Work out the finished part from the listing and answer in its coordinate system (mm). Face numbers are marked on the shaded views. A direction names the side the tool comes from. Round coordinates to 2 decimals unless told otherwise and drop trailing zeros. Write each loop counter-clockwise with the first axis right and the second up, starting at its lowest first coordinate (ties: lowest second). Pieces come first, ordered by that corner, then holes. Notation, with made-up numbers: (24, 45) -> (64, 45) arc R31 ccw to (64, 70) -> close; hole circle Ø9 at (54, -37.5). An arc over 180 degrees is marked (long way). One line per question, with ' | ' between items. Start each with the question number.
Autodesk Fusion 360 part; units mm, degrees
sketch "Sketch1" plane through (0, 0, 0) normal (0, 0, 1) x (1, 0, 0)
  line L0 (0, 0) -> (33, 0)
  line L1 (33, 0) -> (33, -45)
  line L2 (33, -45) -> (0, -45)
  line L3 (0, -45) -> (0, 0)
  circle A0 centre (31, -2) radius 1
  circle A1 centre (2, -2) radius 1
  circle A2 centre (2, -43) radius 1
  circle A3 centre (31, -43) radius 1
  line L4 (34, 1) -> (34, -46)
  line L5 (34, -46) -> (-1, -46)
  line L6 (-1, -46) -> (-1, 1)
  line L7 (-1, 1) -> (34, 1)
  line L8 (36, 3) -> (36, -48)
  line L9 (36, -48) -> (-3, -48)
  line L10 (-3, -48) -> (-3, 3)
  line L11 (-3, 3) -> (36, 3)
  circle A4 centre (31, -2) radius 2
  circle A5 centre (31, -43) radius 2
  circle A6 centre (2, -43) radius 2
  circle A7 centre (2, -2) radius 2
  line L12 (31, -36) -> (2, -36)
  line L13 (2, -36) -> (2, -7)
  line L14 (2, -7) -> (31, -7)
  line L15 (31, -7) -> (31, -36)
extrude "Extrude1" add sketch "Sketch1" along normal blind 20 contours L8 L9 L10 L11 makes body 1
extrude "Extrude2" add sketch "Sketch1" along normal blind 4 separate body contours A7 | A4 | A6 | A5 makes body 2 at (32.9975, -43.0997, 1.3333) makes body 3 at (0.6766, -41.5004, 2.6667) makes body 4 at (32.9975, -2.0997, 1.3333) makes body 5 at (3.9975, -2.0997, 1.3333)
extrude "Extrude3" add sketch "Sketch1" against normal blind 1 contours L0 L3 A7 | L0 L1 L2 L3 A4 A5 A6 A7 | A7 | L0 L1 A4 | A4 | L2 L3 A6 | A6 | A5 | L1 L2 A5 | A0 | A1 | A2 | A3 | L4 L5 L6 L7 | L8 L9 L10 L11 bodies 1 2 3 4 5
extrude "Extrude4" cut 1 faces at (35.3333, -30.3333, 20) along direction (0, 0, -1) blind 10 on bodies 1 bodies 1
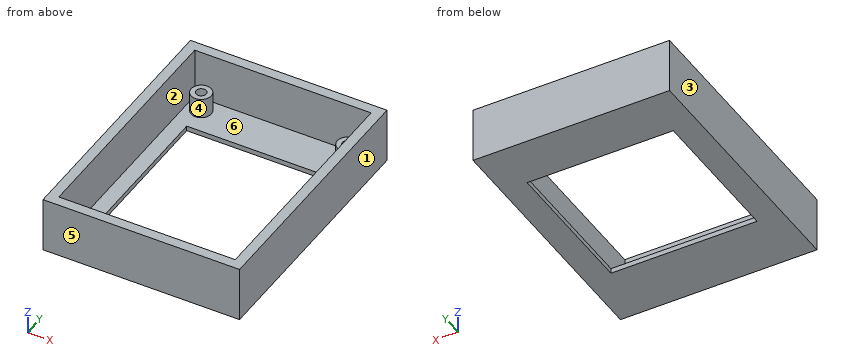
(1) A cutting plane is placed at D-D, the plane z = 6.75. Determine the outline of the cut face in (x, y).
(2) Given pin 1 Ø0.6 at (x, y) = (31, -43) entering from +Z; pin 2 Ø1.2 at (x, y) = (1.5, -1.5) entering from +Z; pin 3 Ø10 at (x, y) = (30, -37) entering from +Z, each flat-ended and moving along its own axis, determine where each tip first touches the part or whether it passes through.
(3) A cutting plane is placed at C-C, the plane x = 19. Determine the outline of the cut face in (y, z), then the cut area to 3 significant figures.
(4) A cutting plane is placed at A-A, the plane y = -29. Determine the outline of the cut face in (x, z).
(5) A cutting plane is placed at B-B, the plane z = 2.75. Count the separate pieces of the cut face and the enclosed holes in it, then the cut area to 3 significant figures.
(6) The mould has two halves that part along X. Classify the marked faces 3, 4, 5 and 6: +X half, -X half, draft (parallel to the pull), parting line (faces both ways), or undercut.
(7) Consider L1, parallel to Y at x = 31, z = 2.4; L2, parallel to X at y = -35, z = 3; L3, parallel to Y at x = 30, z = 4.25. Determine where each line is inside the solid, lowest interval first.
(8) For the marked faces 1 and 2, determine the directions among +Z, -Z, +X, -X, +Y, -Y from which every point of the face is accessible in a straight line to the end or side of a thin tool.
Returned:
1) outline: (-3, -48) -> (36, -48) -> (36, 3) -> (-3, 3) -> close; hole (-1, -46) -> (34, -46) -> (34, 1) -> (-1, 1) -> close
2) pin 1: z = 0 | pin 2: z = 4 | pin 3: z = 10
3) outline: (-48, -1) -> (-36, -1) -> (-36, 0) -> (-46, 0) -> (-46, 10) -> (-48, 10) -> close; (-7, -1) -> (3, -1) -> (3, 10) -> (1, 10) -> (1, 0) -> (-7, 0) -> close | area: 62.0 mm2
4) outline: (-3, -1) -> (2, -1) -> (2, 0) -> (-1, 0) -> (-1, 10) -> (-3, 10) -> close; (31, -1) -> (36, -1) -> (36, 10) -> (34, 10) -> (34, 0) -> (31, 0) -> close
5) separate pieces: 5 | enclosed holes: 5 | area: 382 mm2
6) face 3: -X half | face 4: undercut | face 5: draft | face 6: undercut
7) L1: -48 to -46, -45 to -44, -42 to -41, -4 to -3, -1 to 0, 1 to 3 | L2: -3 to -1, 34 to 36 | L3: -48 to -46, 1 to 3
8) face 1: +Z, -Z, +X, +Y, -Y | face 2: +Z
